Solid Edge part; units mm, degrees
sketch "Sketch1" plane through (0, 0, 0) normal (0, 0, 1) x (1, 0, 0)
  line L0 (30, 22.5) -> (-30, 22.5)
  line L1 (-30, 22.5) -> (-30, -22.5)
  line L2 (-30, -22.5) -> (30, -22.5)
  line L3 (30, -22.5) -> (30, 22.5)
extrude "Protrusion1" add sketch "Sketch1" along normal blind 25
sketch "Sketch2" plane through (0, -22.5, 12.5) normal (0, -1, 0) x (1, 0, 0)
  line L0 (7.5, -4.5) -> (-7.5, -4.5)
  line L1 (-7.5, -4.5) -> (-7.5, -9.5)
  line L2 (-7.5, -9.5) -> (7.5, -9.5)
  line L3 (7.5, -9.5) -> (7.5, -4.5)
  dimension "D1" = 7.5
  dimension "D2" = 7.5
extrude "ExtrudedCutout_1" cut sketch "Sketch2" against normal blind 70.2135
sketch "Sketch3" plane through (-30, 0, 12.5) normal (-1, 0, 0) x (0, -1, 0)
  line L0 (-5, -9.5) -> (5, -9.5)
  line L1 (5, -9.5) -> (5, -4.5)
  line L2 (5, -4.5) -> (-5, -4.5)
  line L3 (-5, -4.5) -> (-5, -9.5)
  dimension "D1" = 5
  dimension "D2" = 5
extrude "ExtrudedCutout_2" cut sketch "Sketch3" against normal blind 138.2134
fillet "Round_2" radius 2.5 16 edges at (-18.75, 5, 3) (-18.75, 5, 8) (-18.75, -5, 8) (-18.75, -5, 3) (18.75, 5, 3) (18.75, 5, 8) (18.75, -5, 8) (18.75, -5, 3) (7.5, -13.75, 8) (-7.5, -13.75, 8) (-7.5, -13.75, 3) (7.5, -13.75, 3) (7.5, 13.75, 3) (7.5, 13.75, 8) (-7.5, 13.75, 3) (-7.5, 13.75, 8)
sketch "Sketch4" plane through (0, 0, 25) normal (0, 0, 1) x (1, 0, 0)
  circle A0 centre (-18, 0) radius 6
extrude "ExtrudedCutout_3" cut sketch "Sketch4" against normal blind 20.7766
fillet "Round_3" radius 1 12 edges at (0, -22.5, 25) (-30, 0, 25) (-30, -22.5, 12.5) (30, -22.5, 12.5) (30, 0, 25) (0, 22.5, 25) (-30, 22.5, 12.5) (0, 22.5, 0) (-30, 0, 0) (0, -22.5, 0) (30, 0, 0) (30, 22.5, 12.5)
sketch "Sketch5" plane through (0, -22.5, 12.5) normal (0, -1, 0) x (1, 0, 0)
  line L0 (-30, 9.5) -> (31.8803, 9.5)
  line L1 (-30, 9.5) -> (-37.6022, -5.1016)
  line L2 (-37.6022, -5.1016) -> (-25.716, -26.0845)
  line L3 (-25.716, -26.0845) -> (61.3689, -24.1439)
  line L4 (61.3689, -24.1439) -> (49.3614, 9.5)
  line L5 (49.3614, 9.5) -> (31.8803, 9.5)
extrude "ExtrudedCutout_4" cut sketch "Sketch5" against normal blind 86.4781
sketch "Sketch6" plane through (0, 0, 22) normal (0, 0, -1) x (1, 0, 0)
  line L0 (-26, -18.5) -> (26, -18.5)
  line L1 (26, -18.5) -> (26, 18.5)
  line L2 (26, 18.5) -> (-26, 18.5)
  line L3 (-26, 18.5) -> (-26, -18.5)
  line L4 (-27.5, -20) -> (27.5, -20)
  line L5 (27.5, -20) -> (27.5, 20)
  line L6 (27.5, 20) -> (-27.5, 20)
  line L7 (-27.5, 20) -> (-27.5, -20)
  dimension "D1" = 26
  dimension "D2" = 26
  dimension "D3" = 27.5
  dimension "D4" = 27.5
extrude "ExtrudedProtrusion_2" add sketch "Sketch6" along normal blind 1.5
Geometry: final body of the model. Coordinates: model frame, mm. A direction names the side the tool comes from. Coordinates: 2 decimals unless noted, no trailing zeros. Order: outer loops, then holes, each group sorted by start corner. A loop starts at its lowest first (then second) coordinate and runs counter-clockwise, first axis right, second up. Notation, with made-up numbers: (48.5, 86.25) - (78.5, 86.25) arc R27 cw to (78.5, 120.25) - close; hole circle Ø4 at (27, 3.5). An arc over 180 degrees is marked (long way). Return JSON: item names as keys, results as strings. Group by question number.
1. Set-up query: faces 1 (the face through (26, 0, 21)), 2 (the face through (-27.5, 0, 21)), 3 (the face through (0, -20, 21)). Return all of +Z, -Z, +X, -X, +Y, -Y with unobstructed straight access to the full face (end or side cutting, diameter ignored); none if empty.
2. Pull-direction query (Y, two-part tool) for faces 4 (the face through (-30, 0, 23)), 5 (the face through (-26, 0, 21)), 6 (the face through (0, 20, 21)); classes: pulls with the +Y half, pulls with the -Y half, needs draft (parallel to the pull), parting line crosses it, or undercut.
3. Cut plane B-B (x = -18). Output: boundary loops of the cut face in (y, z).
4. Cut plane D-D (y = 11.5). Output: boundary loops of the cut face in (x, z).
5. Material intervals for line 1 along X through (y, z) = (-3, 21); line 2 along Y through (x, z) = (-11, 21.75); line 3 along Y through (x, z) = (-18, 23.5), sorted ascending. Write a range as [from, to].
6. Pin query (flat end, axial travel): pin 1 (1.2 mm diameter, centred on y = -2, z = 21, fed in from -X); pin 2 (3 mm diameter, centred on x = -4.5, y = 8.5, fed in from -Z); pin 3 (0.8 mm diameter, centred on x = 10, z = 21.5, fed in from +Y). Return the tip coordinate at first contact, or that it passes through.
7. Cut plane A-A (y = 0). Output: boundary loops of the cut face in (x, z).
8. Cut plane C-C (z = 23). Output: boundary loops of the cut face in (x, y).
Resolved:
{
 "1": {"face 1": "-Z", "face 2": "-Z, -X, +Y, -Y", "face 3": "-Z, +X, -X, -Y"},
 "2": {"face 4": "needs draft", "face 5": "undercut", "face 6": "pulls with the +Y half"},
 "3": {"outline": "(-22.5, 22) - (-20, 22) - (-20, 20.5) - (-18.5, 20.5) - (-18.5, 22) - (-6, 22) - (-6, 25) - (-21.5, 25) arc R1 ccw to (-22.5, 24) - close; (6, 22) - (18.5, 22) - (18.5, 20.5) - (20, 20.5) - (20, 22) - (22.5, 22) - (22.5, 24) arc R1 ccw to (21.5, 25) - (6, 25) - close"},
 "4": {"outline": "(-30, 22) - (-27.5, 22) - (-27.5, 20.5) - (-26, 20.5) - (-26, 22) - (26, 22) - (26, 20.5) - (27.5, 20.5) - (27.5, 22) - (30, 22) - (30, 24) arc R1 ccw to (29, 25) - (-29, 25) arc R1 ccw to (-30, 24) - close"},
 "5": {"line 1": "x = [-27.5, -26], [26, 27.5]", "line 2": "y = [-20, -18.5], [18.5, 20]", "line 3": "y = [-22.5, -6], [6, 22.5]"},
 "6": {"pin 1": "stops at x = -27.5", "pin 2": "stops at z = 22", "pin 3": "stops at y = 20"},
 "7": {"outline": "(-30, 22) - (-27.5, 22) - (-27.5, 20.5) - (-26, 20.5) - (-26, 22) - (-24, 22) - (-24, 25) - (-29, 25) arc R1 ccw to (-30, 24) - close; (-12, 22) - (26, 22) - (26, 20.5) - (27.5, 20.5) - (27.5, 22) - (30, 22) - (30, 24) arc R1 ccw to (29, 25) - (-12, 25) - close"},
 "8": {"outline": "(-30, -21.5) arc R1 ccw to (-29, -22.5) - (29, -22.5) arc R1 ccw to (30, -21.5) - (30, 21.5) arc R1 ccw to (29, 22.5) - (-29, 22.5) arc R1 ccw to (-30, 21.5) - close; hole circle Ø12 at (-18, 0)"}
}
